For this review, take the finished solid that the model builds, in its own axes (mm). A direction names the side the tool comes from. Give positions to 0.01 mm unless a question says otherwise; leave off trailing zeros. Loops run counter-clockwise (first coordinate to the right, second up) from the corner with the lowest first, then second, coordinate; pieces in that order, holes last. Notation, with made-up numbers: M 75,25.25 L 99,25.25 A17 ccw 99,47.25 Z; hole C 9,-24 d10. An arc over 180 degrees is marked long. Use CSV: the item, a comma, the result in double quotes. Start each with the question number.
1. Take a section at C-C, the plane x = 21.5. Write out the cut boundary in (y, z), and give its area (3 significant figures).
2. Take a section at A-A, the plane x = 4. Write out the cut boundary in (y, z).
3. Take a section at B-B, the plane y = 5. Write out the cut boundary in (x, z).
4. The part is to be moulded in two halves that separate along X. For faces 1 (the face through (38, 1.7, -7)), 2 (the face through (5.386, 4.425, 0.986)), 3 (the face through (19, 16, 2)), 4 (the face through (27.3, 0.99, -13.15)), say which applies: pulls with the +X half, pulls with the -X half, needs draft (parallel to the pull), parting line crosses it, or undercut.
5. Insertion check: P1, Ø2.5, axis at x = 4, y = 5, coming from the +Z side; P2, Ø3, axis at x = 14, y = 28, coming from the -Z side; P3, Ø5, axis at x = 26, z = -10.5, coming from the +Y side. Each pin has a flat end and moves straight along its axis. Give the tip position at first contact, or say it passes through.
6. Take a section at D-D, the plane z = -17.5. Write out the cut boundary in (x, y), and give its area (3 significant figures).
7. Tool access review of faces 5 (the face through (32.8, 4.1, 1)), 6 (the face through (19, 17, 0)): name each direction out of +Z, -Z, +X, -X, +Y, -Y from which nothing blocks a thin tool from reaching the whole face with its end or side.
8. To check wall thickness, follow line 1 (Y direction, x = 4, z = 1.3); line 2 (X direction, y = 28, z = 0.5); line 3 (Z direction, x = 15, y = 7.5). State the ranges of each line that lie inside material, in increasing order. Write a range as [from, to].
from build123d import *

# Parameters (mm, degrees)
SKETCH_3_W               = 38
SKETCH_3_H               = 32
EXTRUDE_330_DEPTH        = 2
SKETCH_4_W               = 38
SKETCH_4_H               = 32
EXTRUDE_444_DEPTH        = 2
CUT_EXTRUDE_1_DEPTH      = 59.034472514
CUT_EXTRUDE_1_DEPTH_BACK = 59.034472514
SKETCH_5_R               = 1.5
CUT_EXTRUDE_2_DEPTH      = 59.034472514
CUT_EXTRUDE_2_DEPTH_BACK = 59.034472514
SKETCH_6_R               = 6.656
SKETCH_6_R_2             = 0.8448


with BuildPart() as part:
    # 草图3 → Extrude 330 (new body)
    with BuildSketch(Plane.XY):
        with Locations((19, 16)):
            Rectangle(SKETCH_3_W, SKETCH_3_H)
    extrude(amount=EXTRUDE_330_DEPTH)

    # 草图4 → Extrude 444 (add)
    with BuildSketch(Plane(origin=(0, 0, 0), x_dir=(1, 0, 0), z_dir=(0, 1, 0))):
        with Locations((19, 14)):
            Rectangle(SKETCH_4_W, SKETCH_4_H)
    extrude(amount=EXTRUDE_444_DEPTH)

    # 草图5 → 切除-拉伸1 (cut, two sides: drawn at the far end of the back side and taken through both)
    with BuildSketch(Plane.XY.offset(-CUT_EXTRUDE_1_DEPTH_BACK)):
        with Locations((4, 5)):
            Circle(SKETCH_5_R)
        with Locations((4, 28)):
            Circle(SKETCH_5_R)
        with Locations((34, 5)):
            Circle(SKETCH_5_R)
        with Locations((34, 28)):
            Circle(SKETCH_5_R)
    extrude(amount=CUT_EXTRUDE_1_DEPTH + CUT_EXTRUDE_1_DEPTH_BACK, mode=Mode.SUBTRACT)

    # 草图6 → 切除-拉伸2 (cut, two sides: drawn at the far end of the back side and taken through both)
    with BuildSketch(Plane(origin=(0, 0, 0), x_dir=(1, 0, 0), z_dir=(0, 1, 0)).offset(-CUT_EXTRUDE_2_DEPTH_BACK)):
        with Locations(Location((18.664843729, 13.928843729, 0), (0, 0, 270))):
            Circle(SKETCH_6_R)
        with Locations(Location((9.704843729, 13.928843729, 0), (0, 0, 270))):
            Circle(SKETCH_6_R_2)
        with Locations(Location((18.664843729, 22.888843729, 0), (0, 0, 270))):
            Circle(SKETCH_6_R_2)
        with Locations(Location((27.624843729, 13.928843729, 0), (0, 0, 270))):
            Circle(SKETCH_6_R_2)
        with Locations(Location((18.664843729, 4.968843729, 0), (0, 0, 270))):
            Circle(SKETCH_6_R_2)
    extrude(amount=CUT_EXTRUDE_2_DEPTH + CUT_EXTRUDE_2_DEPTH_BACK, mode=Mode.SUBTRACT)


solid = part.part
Result set:
1,outline,"M 0,-30 L 2,-30 L 2,-19.95 L 0,-19.95 Z; M 0,-7.91 L 2,-7.91 L 2,0 L 32,0 L 32,2 L 0,2 Z"
1,area,"99.9 mm2"
2,outline,"M 0,-30 L 2,-30 L 2,0 L 3.5,0 L 3.5,2 L 0,2 Z; M 6.5,0 L 26.5,0 L 26.5,2 L 6.5,2 Z; M 29.5,0 L 32,0 L 32,2 L 29.5,2 Z"
3,outline,"M 0,0 L 2.5,0 L 2.5,2 L 0,2 Z; M 5.5,0 L 32.5,0 L 32.5,2 L 5.5,2 Z; M 35.5,0 L 38,0 L 38,2 L 35.5,2 Z"
4,face 1,"pulls with the +X half"
4,face 2,"undercut"
4,face 3,"needs draft"
4,face 4,"undercut"
5,P1,"through"
5,P2,"z = 0"
5,P3,"y = 2"
6,outline,"M 0,0 L 13.05,0 L 13.05,2 L 0,2 Z; M 24.28,0 L 38,0 L 38,2 L 24.28,2 Z"
6,area,"53.5 mm2"
7,face 5,"+Z, -Z"
7,face 6,"-Z, +X, -X, +Y"
8,line 1,"[0, 3.5], [6.5, 26.5], [29.5, 32]"
8,line 2,"[0, 2.5], [5.5, 32.5], [35.5, 38]"
8,line 3,"[0, 2]"
